Drawing for the job (mm, zero at the part's lowest x, y, z). Round coordinates to 2 decimals unless told otherwise and drop trailing zeros. Write each loop counter-clockwise with the first axis right and the second up, starting at its lowest first coordinate (ties: lowest second). Pieces come first, ordered by that corner, then holes. Notation, with made-up numbers: (54.25, -36) - (112.25, -36) arc R16 ccw to (112.25, -17) - close; hole circle Ø3 at (80.5, -37). An arc over 180 degrees is marked (long way). Answer in a Markdown table with one row per item.
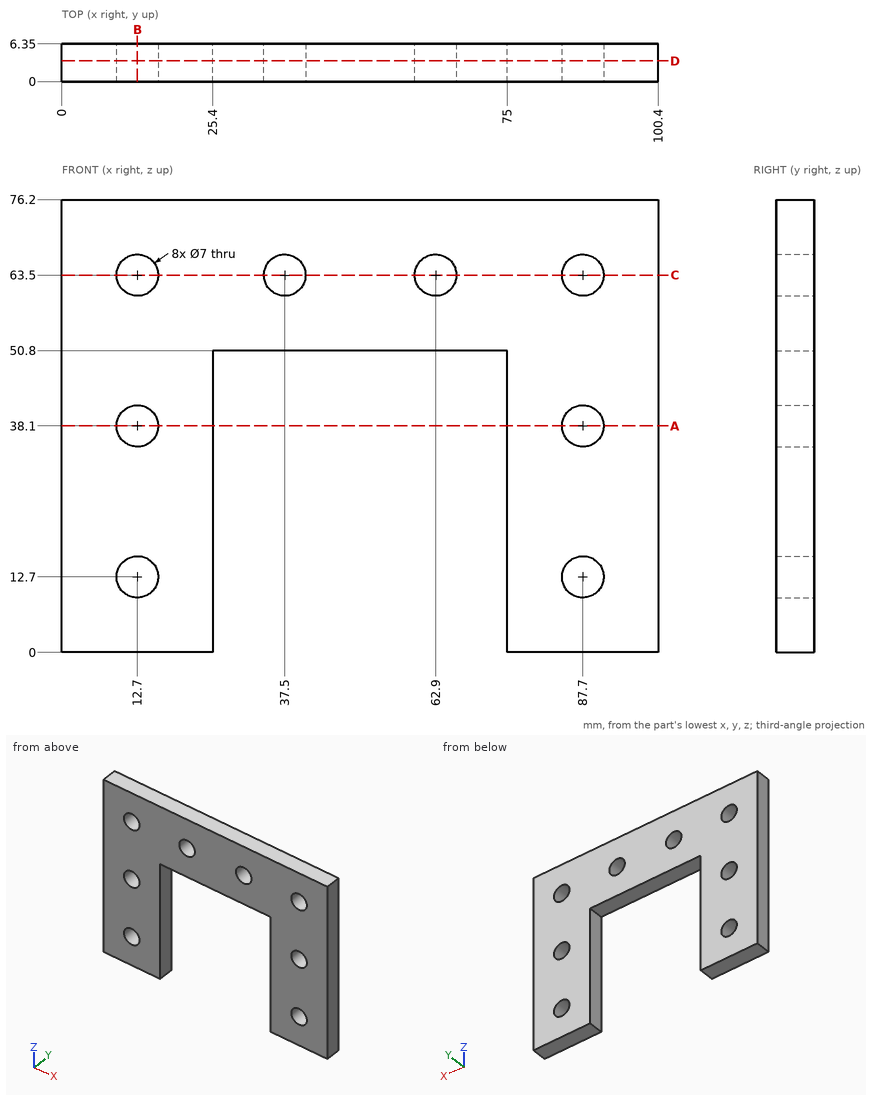
Q1. Flat gauge pin, fed straight in: pin 1 (2 mm diameter, centred on x = 72, y = 5, fed in from -Z). Where does the tip first touch, or does it go through?
Computed:
| item | result |
|---|---|
| pin 1 | stops at z = 50.8 |
Q2. Saw through at B-B on x = 12.7. List the corners of the cut face in (y, z).
Computed:
| item | result |
|---|---|
| outline | (0, 0) - (6.35, 0) - (6.35, 9.2) - (0, 9.2) - close; (0, 16.2) - (6.35, 16.2) - (6.35, 34.6) - (0, 34.6) - close; (0, 41.6) - (6.35, 41.6) - (6.35, 60) - (0, 60) - close; (0, 67) - (6.35, 67) - (6.35, 76.2) - (0, 76.2) - close |
Q3. Saw through at A-A on z = 38.1. List the corners of the cut face in (x, y), then the cut area to 3 significant figures.
Computed:
| item | result |
|---|---|
| outline | (0, 0) - (9.2, 0) - (9.2, 6.35) - (0, 6.35) - close; (16.2, 0) - (25.4, 0) - (25.4, 6.35) - (16.2, 6.35) - close; (75, 0) - (84.2, 0) - (84.2, 6.35) - (75, 6.35) - close; (91.2, 0) - (100.4, 0) - (100.4, 6.35) - (91.2, 6.35) - close |
| area | 234 mm2 |
Q4. Saw through at C-C on z = 63.5. List the corners of the cut face in (x, y), then the cut area to 3 significant figures.
Computed:
| item | result |
|---|---|
| outline | (0, 0) - (9.2, 0) - (9.2, 6.35) - (0, 6.35) - close; (16.2, 0) - (34, 0) - (34, 6.35) - (16.2, 6.35) - close; (41, 0) - (59.4, 0) - (59.4, 6.35) - (41, 6.35) - close; (66.4, 0) - (84.2, 0) - (84.2, 6.35) - (66.4, 6.35) - close; (91.2, 0) - (100.4, 0) - (100.4, 6.35) - (91.2, 6.35) - close |
| area | 460 mm2 |
Q5. Drill centre lines: line 1 (Z direction, x = 87.7, y = 3.25); line 2 (X direction, y = 5.25, z = 19.5); line 3 (X direction, y = 0.75, z = 66.5). Where is each one in solid material? Low to high.
Computed:
| item | result |
|---|---|
| line 1 | z = 0 to 9.2, 16.2 to 34.6, 41.6 to 60, 67 to 76.2 |
| line 2 | x = 0 to 25.4, 75 to 100.4 |
| line 3 | x = 0 to 10.9, 14.5 to 35.7, 39.3 to 61.1, 64.7 to 85.9, 89.5 to 100.4 |
Q6. Saw through at D-D on y = 3.5. Count the separate pieces of the cut face and the enclosed holes in it, then the cut area to 3 significant figures.
Computed:
| item | result |
|---|---|
| separate pieces | 1 |
| enclosed holes | 8 |
| area | 4,820 mm2 |
